Design review of the part shown in the three views and the two pictorial views. Dimensions are in mm from the part's minimum x, y and z. A direction names the side the tool comes from. Give positions to 0.01 mm unless a question says otherwise; leave off trailing zeros. Loops run counter-clockwise (first coordinate to the right, second up) from the corner with the lowest first, then second, coordinate; pieces in that order, holes last. Notation, with made-up numbers: (-12.5, -39) - (21.5, -39) arc R18 ccw to (21.5, -12) - close; hole circle Ø1 at (72.25, 3.5). An arc over 180 degrees is marked (long way). Use CSV: the item, a comma, the result in double quotes. Start each with the question number.
1. Take a section at B-B on x = 6.25. Give the boundary of the cut face in (y, z) (1 decimal), plus the area to 3 significant figures.
2. Take a section at C-C on z = 3. Give the boundary of the cut face in (x, y).
3. For the marked faces 1, 2 and 3, list the 3-axis set-ups (+Z, -Z, +X, -X, +Y, -Y) from which the entire face can be reached by the end or side of a thin tool; tool diameter is ignored.
4. Wall thickness on line 1 (Y direction, x = 0.75, z = 13.5); line 2 (Y direction, x = 2.5, z = 8.25): over which ranges is each line inside the solid? List them lowest first.
5. Mouldability with a two-part tool opening along Z and no side actions: class the marked faces 4, 5, 6 and 7 as pulls with the +Z half, pulls with the -Z half, needs draft (parallel to the pull), parting line crosses it, or undercut.
6. For pin 1 (2 mm diameter, centred on x = 8, y = 12.5, fed in from +Z); pin 2 (1.2 mm diameter, centred on x = 7, y = 7, fed in from -Z); pin 3 (1.5 mm diameter, centred on x = 1, y = 6, fed in from +Z), all flat-tipped, find the tip position at first contact; note any pin that passes through.
7. Take a section at A-A on y = 3.5. Give the boundary of the cut face in (x, z), plus the area to 3 significant figures.
8. Take a section at D-D on z = 5.5. Give the boundary of the cut face in (x, y), plus the area to 3 significant figures.
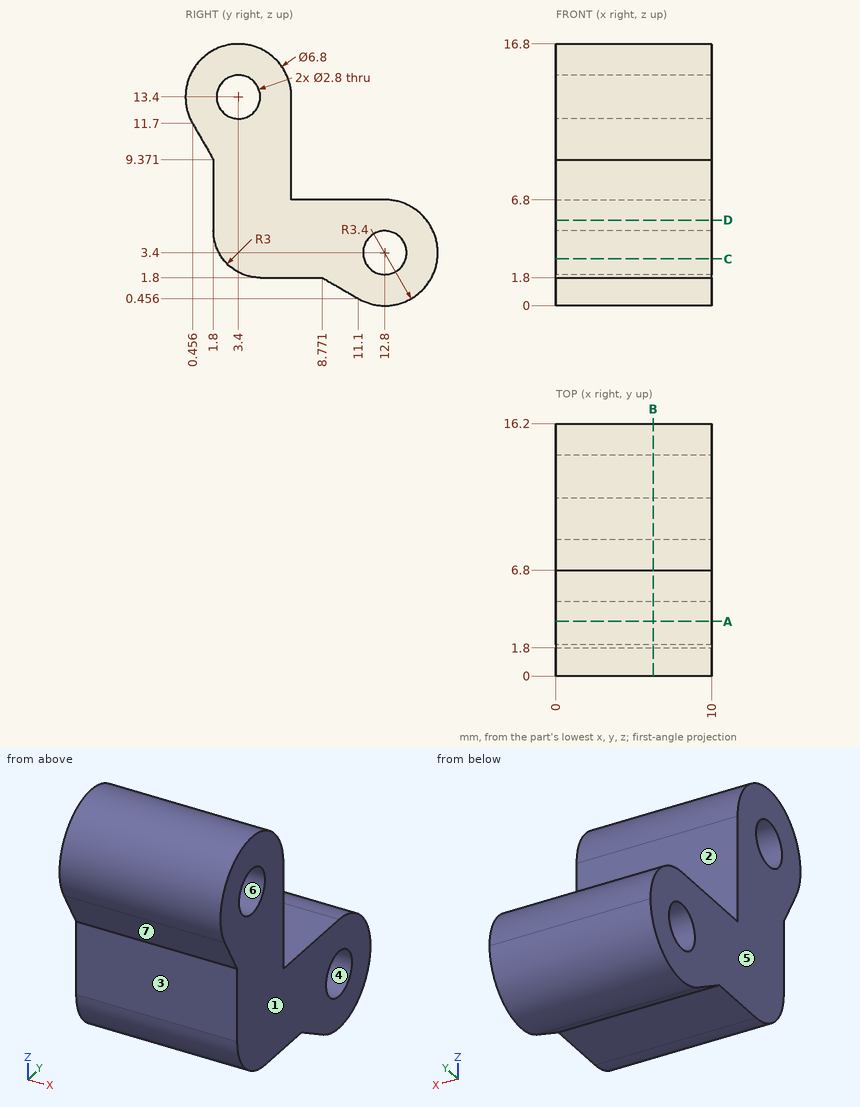
Check result:
1,outline,"(0.5, 11.7) - (1.8, 9.4) - (1.8, 4.8) arc R3 ccw to (4.8, 1.8) - (8.8, 1.8) - (11.1, 0.5) arc R3.4 ccw (long way) to (12.8, 6.8) - (6.8, 6.8) - (6.8, 13.4) arc R3.4 ccw (long way) to start; hole circle Ø2.8 at (3.4, 13.4); hole circle Ø2.8 at (12.8, 3.4)"
1,area,"119 mm²"
2,outline,"(0, 2.4) - (10, 2.4) - (10, 11.46) - (0, 11.46) - close; (0, 14.14) - (10, 14.14) - (10, 16.18) - (0, 16.18) - close"
3,face 1,"+Z, -Z, +X, +Y, -Y"
3,face 2,"+Z, +X, -X, +Y"
3,face 3,"-Z, +X, -X, -Y"
4,line 1,"y = 0 to 2, 4.8 to 6.8"
4,line 2,"y = 1.8 to 6.8"
5,face 4,"undercut"
5,face 5,"needs draft"
5,face 6,"undercut"
5,face 7,"pulls with the -Z half"
6,pin 1,"stops at z = 6.8"
6,pin 2,"stops at z = 1.8"
6,pin 3,"stops at z = 16.25"
7,outline,"(0, 2.1) - (10, 2.1) - (10, 12) - (0, 12) - close; (0, 14.8) - (10, 14.8) - (10, 16.8) - (0, 16.8) - close"
7,area,"119 mm²"
8,outline,"(0, 1.8) - (10, 1.8) - (10, 15.47) - (0, 15.47) - close"
8,area,"137 mm²"
